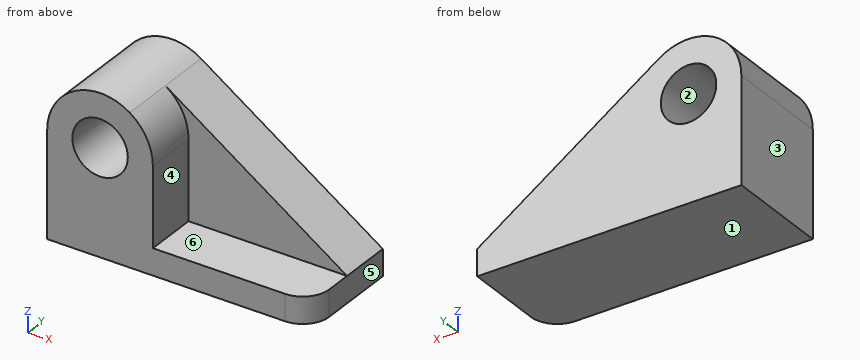
```python
from build123d import *

# Parameters (mm, degrees)
F0_R     = 13.341741
F1_DEPTH = 25.4
F2_R     = 13.341741
F3_DEPTH = 25.4
F4_R     = 12.7


with BuildPart() as f1:
    # F0 (on Front) → F1 (new body)
    with BuildSketch(Plane.XZ):
        with BuildLine():
            Line((49.160112, -31.571778), (-38.202015, 27.56255))
            ThreePointArc((-38.202015, 27.56255), (-64.346148, 28.964821), (-77.839888, 6.528222))
            Line((-77.839888, 6.528222), (-77.839888, -44.271778))
            Line((-77.839888, -44.271778), (49.160112, -44.271778))
            Line((49.160112, -44.271778), (49.160112, -31.571778))
        make_face()
        with Locations((-52.439888, 6.528222)):
            Circle(F0_R, mode=Mode.SUBTRACT)
    extrude(amount=F1_DEPTH)

    # F2 (on face) → F3 (join)
    with BuildSketch(Plane.XZ.offset(25.4)):
        with BuildLine():
            Line((-27.039888, -31.571778), (-27.039888, 6.528222))
            ThreePointArc((-27.039888, 6.528222), (-30.003289, 18.434481), (-38.202015, 27.56255))
            ThreePointArc((-38.202015, 27.56255), (-64.346148, 28.964821), (-77.839888, 6.528222))
            Line((-77.839888, 6.528222), (-77.839888, -31.571778))
            Line((-77.839888, -31.571778), (-77.839888, -44.271778))
            Line((-77.839888, -44.271778), (49.160112, -44.271778))
            Line((49.160112, -44.271778), (49.160112, -31.571778))
            Line((49.160112, -31.571778), (-27.039888, -31.571778))
        make_face()
        with Locations((-52.439888, 6.528222)):
            Circle(F2_R, mode=Mode.SUBTRACT)
    extrude(amount=F3_DEPTH)

    # F4
    f4_edges = [f1.edges().sort_by_distance(p)[0] for p in [
        (49.160112, -50.8, -37.921778),
    ]]
    fillet(f4_edges, radius=F4_R)


solid = f1.part
```
Input: part model. Units: mm. Frame: model coordinates. Face numbers are marked on the shaded views. A direction names the side the tool comes from. Round coordinates to 2 decimals unless told otherwise and drop trailing zeros. Write each loop counter-clockwise with the first axis right and the second up, starting at its lowest first coordinate (ties: lowest second). Pieces come first, ordered by that corner, then holes. Notation, with made-up numbers: M 18.25,42 L 46.25,42 A15 cw 46.25,67 Z; hole C 7,70.5 d10. An arc over 180 degrees is marked long. Write each question's results on one line, items separated by ' | '.
Q1. Section query C-C (z = 3). Return loops of the section in (x, y).
Results:
outline: M -77.84,-50.8 L -65.31,-50.8 L -65.31,0 L -77.84,0 Z; M -39.57,-50.8 L -27.04,-50.8 L -27.04,-25.4 L -1.91,-25.4 L -1.91,0 L -39.57,0 Z
Q2. Section query D-D (y = -41). Return loops of the section in (x, z).
Results:
outline: M -77.84,-44.27 L 48.82,-44.27 L 48.82,-31.57 L -27.04,-31.57 L -27.04,6.53 A25.4 ccw -38.2,27.56 A25.4 ccw -77.84,6.53 Z; hole C -52.44,6.53 d26.68
Q3. Line query: line 1 along Z through (x, y) = (20, -32); line 2 along Z through (x, y) = (-56, -11); line 3 along Y through (x, z) = (-21.5, 3.5). Output: solid intervals per line, ascending.
Results:
line 1: z = -44.27 to -31.57 | line 2: z = -44.27 to -6.33, 19.39 to 31.68 | line 3: y = -25.4 to 0
Q4. Access query for the marked faces 5 and 6. Directions: +Z, -Z, +X, -X, +Y, -Y. A direction counts if a zero-diameter tool reaches every point of the face in a straight line with its end or side. Return the directions, or none.
Results:
face 5: +Z, -Z, +X, +Y, -Y | face 6: +Z, +X, -Y
Q5. Section query B-B (x = -45.5). Return loops of the section in (y, z), and give its area (3 significant figures).
Results:
outline: M -50.8,-44.27 L 0,-44.27 L 0,-4.87 L -50.8,-4.87 Z; M -50.8,17.92 L 0,17.92 L 0,30.96 L -50.8,30.96 Z | area: 2,660 mm^2
Q6. Draft query along X for the marked faces 1, 2, 3 and 4. Return one class per face: released by +X, released by -X, zero draft, split by the parting line, or undercut.
Results:
face 1: zero draft | face 2: undercut | face 3: released by -X | face 4: released by +X
Q7. Section query A-A (y = -34). Return loops of the section in (x, z), and give its area (3 significant figures).
Results:
outline: M -77.84,-44.27 L 49.16,-44.27 L 49.16,-31.57 L -27.04,-31.57 L -27.04,6.53 A25.4 ccw -38.2,27.56 A25.4 ccw -77.84,6.53 Z; hole C -52.44,6.53 d26.68 | area: 4,000 mm^2
Q8. Pin query (flat end, axial travel): P1, Ø10, axis at y = -17, z = 23, coming from the +X side; P2, Ø10, axis at y = -16, z = -1, coming from the +X side; P3, Ø8, axis at x = -12, z = -36, coming from the +Y side; P4, Ø7.5, axis at x = 13.5, y = -36, coming from the +Z side. Return the tip coordinate at first contact, or that it passes through.
Results:
P1: stops at x = -24.07 | P2: stops at x = 11.38 | P3: stops at y = 0 | P4: stops at z = -31.57
